```python
from build123d import *

# Parameters (mm, degrees)
EXTRU_MINCE1_DEPTH      = 183
ESQUISSE8_W             = 75
ESQUISSE8_H             = 65
ENL_V_MAT_EXTRU_2_DEPTH = 1
D_GAGEMENT_M32_D        = 3.4
ENL_V_MAT_EXTRU_3_REACH = 173.369
ESQUISSE15_W            = 25
ESQUISSE15_H            = 35
ENL_V_MAT_EXTRU_4_REACH = 173.364
ESQUISSE16_W            = 35
ESQUISSE16_H            = 25


with BuildPart() as part:
    # Esquisse2 → Extru.-Mince1 (new body)
    with BuildSketch(Plane.XY):
        Polygon((-59.170699115, 35.114), (-24.057682042, 0), (145.942317958, 0), (181.056317958, 35.113017073), (181.763414842, 34.405900395), (146.356523321, -1), (-24.471903803, -1), (-59.877815794, 34.406903116), align=None)
    extrude(amount=EXTRU_MINCE1_DEPTH)

    # Esquisse8 → Enlèv. mat.-Extru.2 (cut)
    with BuildSketch(Plane(origin=(0, 0, 0), x_dir=(1, 0, 0), z_dir=(0, 1, 0))):
        with Locations((60.942317958, -32.5)):
            Rectangle(ESQUISSE8_W, ESQUISSE8_H)
    extrude(amount=-ENL_V_MAT_EXTRU_2_DEPTH, mode=Mode.SUBTRACT)

    # Dégagement M32 (through all)
    with Locations(Plane(origin=(0, 0, 0), x_dir=(-1, 0, 0), z_dir=(0, 1, 0))):
        with Locations((18.357682042, 20), (-140.242317958, 20), (-140.242317958, 163), (18.357682042, 163)):
            Hole(D_GAGEMENT_M32_D / 2)

    # Esquisse15 → Enlèv. mat.-Extru.3 (cut, up to next)
    with BuildSketch(Plane(origin=(-12.73629442, -12.7359379, 0), x_dir=(0, 0, 1), z_dir=(-0.707116678, -0.707096884, 0)), mode=Mode.PRIVATE) as enl_v_mat_extru_3_sk1:
        with Locations((12.5, 49.169112012)):
            Rectangle(ESQUISSE15_W, ESQUISSE15_H)
    enl_v_mat_extru_3_tool1 = extrude(enl_v_mat_extru_3_sk1.sketch, amount=-ENL_V_MAT_EXTRU_3_REACH, mode=Mode.PRIVATE) & part.part
    add(enl_v_mat_extru_3_tool1.solids().sort_by_distance((-47.50362, 22.032361, 12.5))[0], mode=Mode.SUBTRACT)

    # Esquisse16 → Enlèv. mat.-Extru.4 (cut, up to next)
    with BuildSketch(Plane(origin=(73.676213194, -73.678275628, 0), x_dir=(0.707116678, 0.707096884, 0), z_dir=(0.707096884, -0.707116678, 0)), mode=Mode.PRIVATE) as enl_v_mat_extru_4_sk1:
        with Locations((135.356247065, 12.5)):
            Rectangle(ESQUISSE16_W, ESQUISSE16_H)
    enl_v_mat_extru_4_tool1 = extrude(enl_v_mat_extru_4_sk1.sketch, amount=-ENL_V_MAT_EXTRU_4_REACH, mode=Mode.PRIVATE) & part.part
    add(enl_v_mat_extru_4_tool1.solids().sort_by_distance((169.388873, 22.031705, 12.5))[0], mode=Mode.SUBTRACT)


solid = part.part
```
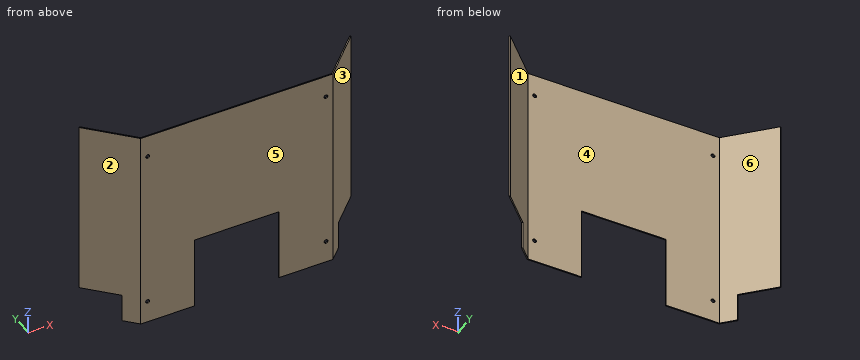
The listing builds one solid part. Answer for the finished solid, in the listing's coordinates (mm). Face numbers are marked on the shaded views. A direction names the side the tool comes from. Round coordinates to 2 decimals unless told otherwise and drop trailing zeros. Loops run counter-clockwise (first coordinate to the right, second up) from the corner with the lowest first, then second, coordinate; pieces in that order, holes last.
Q1. Section D-D, the plane x = 72 is taken. Determine the outline of the cut face in (y, z), then the cut area to 3 significant figures.
Q2. Section A-A, the plane z = 117 is taken. Determine the outline of the cut face in (x, y).
Q3. Find the intervals of material crossed by line 1 (X direction, y = -0.65, z = 163); line 2 (Y direction, x = -18, z = 103); line 3 (X direction, y = 3, z = 36), in increasing order.
Q4. Section B-B, the plane y = 5 is taken. Determine the outline of the cut face in (x, z).
Q5. Which of the six approach directions +Z, -Z, +X, -X, +Y, -Y give full straight-line access (tool end or side, diameter ignored) to the marked faces 5 and 6?
Q6. Section C-C, the plane x = 119 is taken. Determine the outline of the cut face in (y, z).
Q7. Given pin 1 Ø12.5 at (x, y) = (-45, 22.5) entering from -Z; pin 2 Ø2 at (x, z) = (-18.36, 163) entering from +Y; pin 3 Ø12 at (y, z) = (3.5, 31.5) entering from +X; pin 4 Ø1.5 at (y, z) = (7.5, 83) entering from -X, each flat-ended and moving along its own axis, determine where each tip first touches the part or whether it passes through.
Q8. For a pull along X with two mould halves and no side action, classify the marked faces 1, 2, 3 and 4 as released by +X, released by -X, zero draft, split by the parting line, or undercut.
Completed:
1. outline: (-1, 65) - (0, 65) - (0, 183) - (-1, 183) - close
1. area: 118 mm2
2. outline: (-59.88, 34.41) - (-24.47, -1) - (146.36, -1) - (181.76, 34.41) - (181.06, 35.11) - (145.94, 0) - (-24.06, 0) - (-59.17, 35.11) - close
3. line 1: x = -24.82 to -20.06, -16.66 to 138.54, 141.94 to 146.71
3. line 2: y = -1 to 0
3. line 3: x = -28.47 to -27.06, 148.94 to 150.36
4. outline: (-30.47, 0) - (-29.06, 0) - (-29.06, 183) - (-30.47, 183) - close; (150.94, 0) - (152.36, 0) - (152.36, 183) - (150.94, 183) - close
5. face 5: +Z, -Z, +X, -X, -Y
5. face 6: +Z, -Z, +Y
6. outline: (-1, 0) - (0, 0) - (0, 183) - (-1, 183) - close
7. pin 1: stops at z = 25
7. pin 2: passes through
7. pin 3: stops at x = 156.86
7. pin 4: stops at x = -33.72
8. face 1: undercut
8. face 2: released by -X
8. face 3: released by +X
8. face 4: undercut
